The listing builds one solid part. Answer for the finished solid, in the listing's coordinates (mm). Coordinates: 2 decimals unless noted, no trailing zeros. Loops run counter-clockwise (first coordinate to the right, second up) from the corner with the lowest first, then second, coordinate; pieces in that order, holes last. Notation, with made-up numbers: M 21,-18.5 L 61,-18.5 A30 ccw 61,15.5 Z; hole C -36.75,-12 d9. An arc over 180 degrees is marked long. Return JSON: item names as keys, results as strings. Group by question number.
1. Straight lines are drawn through the part: L1, parallel to X at y = 20, z = 6; L2, parallel to Y at x = -20, z = 5.5; L3, parallel to X at y = 16.5, z = 1. For each, find the intervals that lie inside material, in ascending order. Write a range as from..to.
2. Given P1, Ø3.5, axis at x = -24.5, y = 20, coming from the -Z side, flat-ended and moving along its own axis, determine where the tip first touches the part or whether it passes through.
3. Section A-A (x = -20) is taken. Write down the section's boundary in (y, z), then the cut area to 3 significant figures.
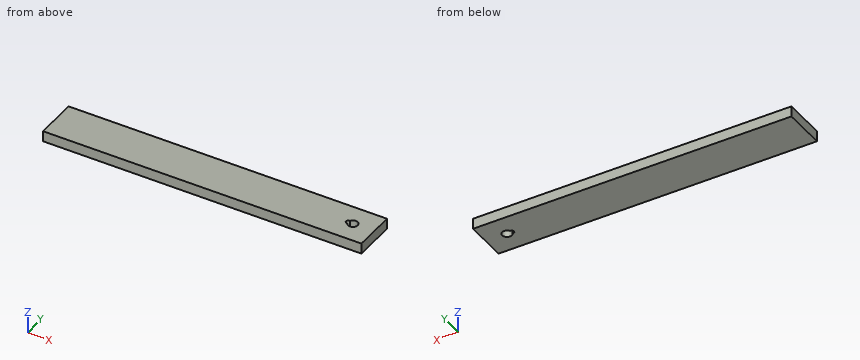
Autodesk Inventor part; units mm, degrees
ref_plane "YZ Plane" through (0, 0, 0) normal (1, 0, 0) x (0, 1, 0)
ref_plane "XZ Plane" through (0, 0, 0) normal (0, 1, 0) x (-1, 0, 0)
ref_plane "XY Plane" through (0, 0, 0) normal (0, 0, 1) x (1, 0, 0)
sketch "Skizze1" plane through (0, 0, 0) normal (0, 0, 1) x (1, 0, 0)
  line L0 (0, 40) -> (-300, 40)
  line L1 (-300, 40) -> (-300, 0)
  line L2 (-300, 0) -> (0, 0)
  line L3 (0, 0) -> (0, 40)
  line L4 (-360, 0) -> (60, 0)
  line L5 (0, -8) -> (0, 48)
  dimension "d0" = 300
  dimension "d1" = 40
extrude "Extrusion1" add sketch "Skizze1" along normal blind 10
sketch "Skizze2" plane through (0, 0, 0) normal (0, 0, -1) x (-1, 0, 0)
  line L0 (0, 40) -> (300, 40)
  line L1 (0, 0) -> (0, 40)
  point P0 (20, 20)
  dimension "d4" = 20
  dimension "d5" = 20
hole "Bohrung1" at (-20, 20, 0) direction (0, 0, 1) diameter 9 end through all
sketch "Skizze3" plane through (0, 0, 0) normal (0, 0, -1) x (-1, 0, 0)
  circle A0 centre (20, 20) radius 4.5
  line L0 (0, 40) -> (300, 40)
  line L1 (20, 20) -> (24.5, 20)
  circle A1 centre (24.5, 20) radius 2
  point P0 (24.0556, 18.05)
  point P1 (24.0556, 21.95)
  dimension "d13" = 4
extrude "Extrusion2" cut sketch "Skizze3" against normal blind 10 contours A0 A1 picked at (25.084, 19.4875)
properties part number "Hebel_camera" material "Holz (Eiche)"
Worked out:
{
 "1": {"L1": "-300..-26.5, -15.5..0", "L2": "0..15.5, 24.5..40", "L3": "-300..-22.83, -17.17..0"},
 "2": {"P1": "through"},
 "3": {"outline": "M 0,0 L 15.5,0 L 15.5,10 L 0,10 Z; M 24.5,0 L 40,0 L 40,10 L 24.5,10 Z", "area": "310 mm^2"}
}
